Can you work these out from the model? Positions are in its coordinate system, mm. A direction names the side the tool comes from. Coordinates: 2 decimals unless noted, no trailing zeros. Loops run counter-clockwise (first coordinate to the right, second up) from the corner with the lowest first, then second, coordinate; pieces in that order, holes last. Notation, with made-up numbers: (-8, 14) -> (37, 14) arc R7 cw to (37, 24) -> close; hole circle Ø8 at (26.5, 5.25). An arc over 180 degrees is marked (long way). Use one line per item in the form item = value. Start each with the question number.
(1) Imagine slicing it at A-A (z = 5). List the corners of the cut face in (x, y) for me (3 decimals).
(2) Thinking about a two-plate mould opening in Z: for faces 5 (the flat face through (48.17, 6, 5)), 6 (the flat face through (26.9, 4.6, 0)), 7 (the cylindrical face through (50.98, 8.732, 4.087)), which applies, released by +Z, released by -Z, zero draft, split by the parting line, or undercut?
(3) I need wall thicknesses on line 1 (X direction, y = 4.5, z = 7.75); line 2 (X direction, y = 8.25, z = 8.25); line 3 (Y direction, x = 22, z = 4). Which ranges of each line are inside material? Lowest first, please. Write a range as [from, to].
(4) Imagine slicing it at D-D (x = 32.5). List the corners of the cut face in (y, z) for me.
(5) Imagine slicing it at C-C (x = 19). List the corners of the cut face in (y, z) for me, plus the area to 3 significant figures.
(6) On a 3-axis mill with a long thin cutter (end or side, diameter ignored), from which of +Z, -Z, +X, -X, +Y, -Y can I reach the whole of each face in a straight line? I mean faces 1 (the flat face through (36, 2.5, 5)), 2 (the flat face through (23.17, 6, 5)), 3 (the flat face through (50, 7.5, 5)), 4 (the flat face through (56.17, 9, 5)). Say none if no direction works.
(7) I'm going to push flat-ended pins straight in: pin 1 (2 mm diameter, centred on y = 1.5, z = 2.5, fed in from -X); pin 2 (1.8 mm diameter, centred on y = 6.5, z = 5.5, fed in from -X); pin 3 (2 mm diameter, centred on x = 21, z = 7, fed in from -Y). Where does each tip first touch, or does it pass through?
(8) Imagine slicing it at B-B (z = 7.5). List the corners of the cut face in (x, y) for me (3 decimals), plus the area to 3 significant figures.
```python
from build123d import *

# Parameters (mm, degrees)
PAD_DEPTH       = 10
SKETCH002_R     = 1.5
POCKET_DEPTH    = 10.001
SKETCH003_W     = 2.5
SKETCH003_H     = 10
PAD001_DEPTH    = 8
SKETCH004_R     = 1.5
POCKET001_DEPTH = 2.501
FILLET_R        = 4


with BuildPart() as part:
    # Sketch → Pad (new body)
    with BuildSketch(Plane.XY):
        with BuildLine():
            ThreePointArc((25.669873, 10), (26.447689, 5.961126), (28.669873, 2.5))
            Line((28.669873, 2.5), (42.669873, 2.5))
            ThreePointArc((42.669873, 2.5), (44.892057, 5.961126), (45.669873, 10))
            Line((48.169873, 10), (45.669873, 10))
            Line((48.169873, 0), (48.169873, 10))
            Line((23.169873, 0), (48.169873, 0))
            Line((23.169873, 0), (23.169873, 7.5))
            Line((23.169873, 7.5), (0, 7.5))
            ThreePointArc((0, 7.5), (-1.25, 7.165064), (-2.165064, 6.25))
            ThreePointArc((-4.330127, 10), (-6.495191, 6.25), (-2.165064, 6.25))
            Line((-4.330127, 10), (23.169873, 10))
            Line((25.669873, 10), (23.169873, 10))
        make_face()
    extrude(amount=PAD_DEPTH)

    # Sketch002 → Pocket (cut, through all)
    with BuildSketch(Plane.XY.offset(10)):
        with Locations((-4.330127, 7.5)):
            Circle(SKETCH002_R)
    extrude(amount=-POCKET_DEPTH, mode=Mode.SUBTRACT)

    # Sketch003 (on Face11 of Pocket) → Pad001 (join)
    with BuildSketch(Plane.YZ.offset(48.169873)):
        with Locations((8.75, 5)):
            Rectangle(SKETCH003_W, SKETCH003_H)
    extrude(amount=PAD001_DEPTH)

    # Sketch004 (on Face11 of Pad001) → Pocket001 (cut, through all)
    with BuildSketch(Plane.XZ.offset(-7.5)):
        with Locations((52.169873, 5)):
            Circle(SKETCH004_R)
        with Locations((19.169873, 5)):
            Circle(SKETCH004_R)
    extrude(amount=-POCKET001_DEPTH, mode=Mode.SUBTRACT)

    # Fillet
    fillet_edges = [part.edges().sort_by_distance(p)[0] for p in [
        (48.169873, 0, 5),
        (23.169873, 0, 5),
    ]]
    fillet(fillet_edges, radius=FILLET_R)


solid = part.part
```
Worked out:
q1.outline = (-4.33, 10) arc R2.5 ccw (long way) to (-2.165, 6.25) arc R2.5 cw to (0, 7.5) -> (17.67, 7.5) -> (17.67, 10) -> close; (20.67, 7.5) -> (23.17, 7.5) -> (23.17, 4) arc R4 ccw to (27.17, 0) -> (44.17, 0) arc R4 ccw to (48.17, 4) -> (48.17, 7.5) -> (50.67, 7.5) -> (50.67, 10) -> (45.67, 10) arc R10.875 cw to (42.67, 2.5) -> (28.67, 2.5) arc R10.875 cw to (25.67, 10) -> (20.67, 10) -> close; (53.67, 7.5) -> (56.17, 7.5) -> (56.17, 10) -> (53.67, 10) -> close; hole circle Ø3 at (-4.33, 7.5)
q2.face_5 = zero draft
q2.face_6 = released by -Z
q2.face_7 = undercut
q3.line_1 = [23.17, 27.16], [44.18, 48.17]
q3.line_2 = [-6.71, -5.63], [-3.03, 25.81], [45.53, 56.17]
q3.line_3 = [7.5, 10]
q4.outline = (0, 0) -> (2.5, 0) -> (2.5, 10) -> (0, 10) -> close
q5.outline = (7.5, 0) -> (10, 0) -> (10, 3.51) -> (7.5, 3.51) -> close; (7.5, 6.49) -> (10, 6.49) -> (10, 10) -> (7.5, 10) -> close
q5.area = 17.5 mm2
q6.face_1 = +Z, -Z, +Y
q6.face_2 = +Z, -Z, -Y
q6.face_3 = +Z, -Z, +X, -Y
q6.face_4 = +Z, -Z, +X, +Y, -Y
q7.pin_1 = 23.46
q7.pin_2 = -6.83
q7.pin_3 = 7.5
q8.outline = (-4.33, 10) arc R2.5 ccw (long way) to (-2.165, 6.25) arc R2.5 cw to (0, 7.5) -> (23.17, 7.5) -> (23.17, 4) arc R4 ccw to (27.17, 0) -> (44.17, 0) arc R4 ccw to (48.17, 4) -> (48.17, 7.5) -> (56.17, 7.5) -> (56.17, 10) -> (45.67, 10) arc R10.875 cw to (42.67, 2.5) -> (28.67, 2.5) arc R10.875 cw to (25.67, 10) -> close; hole circle Ø3 at (-4.33, 7.5)
q8.area = 204 mm2
